Read the model definition and answer for the solid it produces. Units are mm, in the model's axes. A direction names the side the tool comes from. Round coordinates to 2 decimals unless told otherwise and drop trailing zeros. Order: outer loops, then holes, each group sorted by start corner. A loop starts at its lowest first (then second) coordinate and runs counter-clockwise, first axis right, second up. Notation, with made-up numbers: M 49,64 L 102,64 A25 ccw 102,93 Z; hole C -11.5,46.25 d4. An arc over 180 degrees is marked long. Answer as CSV lines item,"result".
```python
from build123d import *

# Parameters (mm, degrees)
BOSS_EXTRUDE1_DEPTH = 6.35
SKETCH2_W           = 38.1
SKETCH2_H           = 20
BOSS_EXTRUDE2_DEPTH = 6.35
SKETCH3_R           = 1.175
CUT_EXTRUDE1_DEPTH  = 7.35
SKETCH4_R           = 2.75
CUT_EXTRUDE2_DEPTH  = 7.35


with BuildPart() as part:
    # Sketch1 → Boss-Extrude1 (new body, symmetric)
    with BuildSketch(Plane.XY):
        Polygon((-13.893293336, 0), (13.893293336, 0), (13.893293336, 76.2), (7.543293336, 76.2), (7.543293336, 6.35), (-13.893293336, 6.35), align=None)
    extrude(amount=BOSS_EXTRUDE1_DEPTH, both=True)

    # Sketch2 → Boss-Extrude2 (add)
    with BuildSketch(Plane.ZY.offset(-7.543293336)):
        with Locations((0, 66.2)):
            Rectangle(SKETCH2_W, SKETCH2_H)
    extrude(amount=-BOSS_EXTRUDE2_DEPTH)

    # Sketch3 → Cut-Extrude1 (cut, through all)
    with BuildSketch(Plane(origin=(0, 6.35, 0), x_dir=(1, 0, 0), z_dir=(0, 1, 0))):
        with BuildLine():
            ThreePointArc((2.056706664, 0.65), (1.524137822, 1.673617376), (0.380238611, 1.825))
            ThreePointArc((0.380238611, 1.825), (-0.443293336, 0.65), (0.380238611, -0.525))
            ThreePointArc((0.380238611, -0.525), (1.524137822, -0.373617376), (2.056706664, 0.65))
        make_face()
        with Locations((-8.693293336, 0.65)):
            Circle(SKETCH3_R)
    extrude(amount=-CUT_EXTRUDE1_DEPTH, mode=Mode.SUBTRACT)

    # Sketch4 → Cut-Extrude2 (cut, through all)
    with BuildSketch(Plane.ZY.offset(-7.543293336)):
        with Locations((-10, 66.2)):
            Circle(SKETCH4_R)
        with Locations((10, 66.2)):
            Circle(SKETCH4_R)
    extrude(amount=-CUT_EXTRUDE2_DEPTH, mode=Mode.SUBTRACT)


solid = part.part
```
Item 1: Flat-ended cylindrical pins translate along their axes: pin 1 (10 mm diameter, centred on x = -1, z = 1, fed in from +Y); pin 2 (8 mm diameter, centred on y = 35, z = 13.5, fed in from +X); pin 3 (3 mm diameter, centred on x = 11.5, z = -13.5, fed in from -Y). Find the tip coordinate at first contact, or state that the pin passes through.
Ans:
pin 1,"y = 6.35"
pin 2,"through"
pin 3,"y = 56.2"
Item 2: A tool of negligible diameter and unlimited length cuts with its end or side. For faces 4 (the face through (8, 20, -6.35)), 5 (the face through (11, 56.2, 13)), 6 (the face through (-3, 6.35, 0)), 7 (the face through (0, 0, 2)), from which of +Z, -Z, +X, -X, +Y, -Y can it reach the whole face along a straight path? Write none if from no direction.
Ans:
face 4,"-Z, +X, -X, -Y"
face 5,"+Z, +X, -X, -Y"
face 6,"+Z, -Z, -X, +Y"
face 7,"+Z, -Z, +X, -X, -Y"
Item 3: A cutting plane is placed at D-D, the plane x = -8.75. Determine the outline of the cut face in (y, z), and give its area (3 significant figures).
Ans:
outline,"M 0,-6.35 L 6.35,-6.35 L 6.35,-1.82 L 0,-1.82 Z; M 0,0.52 L 6.35,0.52 L 6.35,6.35 L 0,6.35 Z"
area,"65.7 mm2"
Item 4: A cutting plane is placed at C-C, the plane z = -10. Determine the outline of the cut face in (x, y), and give its area (3 significant figures).
Ans:
outline,"M 7.54,56.2 L 13.89,56.2 L 13.89,63.45 L 7.54,63.45 Z; M 7.54,68.95 L 13.89,68.95 L 13.89,76.2 L 7.54,76.2 Z"
area,"92.1 mm2"
Item 5: Find the intervals of material crossed by probe 1 along X at (y, z) = (2, 0); probe 2 along Y at (x, z) = (9.25, 10); probe 3 along X at (y, z) = (41.5, -2), in increasing order. Write a range as [from, to].
Ans:
probe 1,"[-13.89, -9.67], [-7.71, -0.26], [1.87, 13.89]"
probe 2,"[56.2, 63.45], [68.95, 76.2]"
probe 3,"[7.54, 13.89]"
Item 6: A cutting plane is placed at B-B, the plane y = 66.2. Determine the outline of the cut face in (x, z).
Ans:
outline,"M 7.54,-19.05 L 13.89,-19.05 L 13.89,-12.75 L 7.54,-12.75 Z; M 7.54,-7.25 L 13.89,-7.25 L 13.89,7.25 L 7.54,7.25 Z; M 7.54,12.75 L 13.89,12.75 L 13.89,19.05 L 7.54,19.05 Z"
Item 7: A cutting plane is placed at A-A, the plane x = 11. Determine the outline of the cut face in (y, z), and give its area (3 significant figures).
Ans:
outline,"M 0,-6.35 L 56.2,-6.35 L 56.2,-19.05 L 76.2,-19.05 L 76.2,19.05 L 56.2,19.05 L 56.2,6.35 L 0,6.35 Z; hole C 66.2,-10 d5.5; hole C 66.2,10 d5.5"
area,"1,430 mm2"
Item 8: Determine the mould class of faces 1 (the face through (-9.867, 3.219, -0.702)), 2 (the face through (8, 20, 6.35)), 3 (the face through (13.893, 47, 0)) for opening direction Z: +Z half, -Z half, draft (parallel to the pull), parting line (faces both ways), or undercut.
Ans:
face 1,"undercut"
face 2,"+Z half"
face 3,"draft"
